Can you work these out from the model? Positions are in its coordinate system, mm. Face numbers are marked on the shaded views. A direction names the side the tool comes from. Round coordinates to 2 decimals unless told otherwise and drop trailing zeros. Loops run counter-clockwise (first coordinate to the right, second up) from the corner with the lowest first, then second, coordinate; pieces in that order, holes last. Notation, with made-up numbers: (82.25, -23.5) -> (111.25, -23.5) arc R34 cw to (111.25, 11.5) -> close; hole circle Ø4 at (-3.75, 80.25). An arc over 180 degrees is marked (long way). Write item = value, one per line.
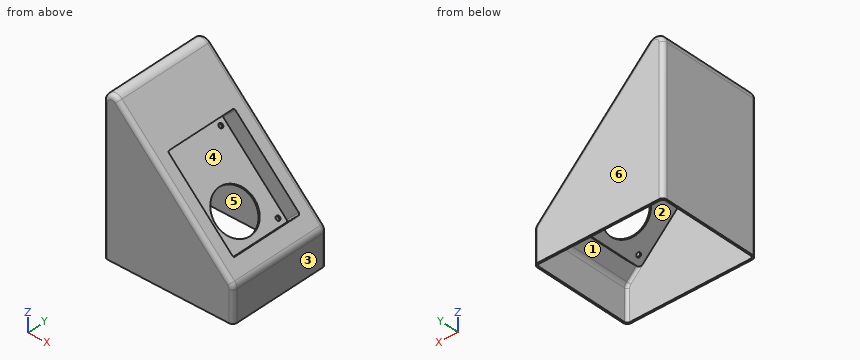
from build123d import *

# Parameters (mm, degrees)
F1_DEPTH = 60
F2_R     = 2.5
F2_R_2   = 25
F3_DEPTH = 20
F4_R     = 5
F5_T     = -2
F6_DEPTH = 25


with BuildPart() as f1:
    # F0 (on Front) → F1 (new body, symmetric)
    with BuildSketch(Plane.XZ):
        with BuildLine():
            Line((-84.0168925865, 63.0011496848), (-84.0168925865, -102.8567146915))
            Line((-84.0168925865, -102.8567146915), (65.9831074135, -102.8567146915))
            Line((65.9831074135, -102.8567146915), (65.9831074135, -66.9988503152))
            ThreePointArc((65.9831074135, -66.9988503152), (65.2219027386, -63.1720159916), (63.0541752254, -59.9277825033))
            Line((63.0541752254, -59.9277825033), (-66.9458247746, 70.0722174967))
            ThreePointArc((-66.9458247746, 70.0722174967), (-77.8437269101, 72.2399450099), (-84.0168925865, 63.0011496848))
        make_face()
    extrude(amount=F1_DEPTH, both=True)

    # F2 (on face) → F3 (cut)
    with BuildSketch(Plane(origin=(1.563196361, 0, 1.563196361), x_dir=(0.7071067812, 0, -0.7071067812), z_dir=(0.7071067812, 0, 0.7071067812))):
        with BuildLine():
            ThreePointArc((69.6613762736, 40.7), (69.0755898359, 42.1142135624), (67.6613762736, 42.7))
            Line((67.6613762736, 42.7), (-35.8386237264, 42.7))
            ThreePointArc((-35.8386237264, 42.7), (-37.2528372888, 42.1142135624), (-37.8386237264, 40.7))
            Line((-37.8386237264, 40.7), (-37.8386237264, -40.7))
            ThreePointArc((-37.8386237264, -40.7), (-37.2528372888, -42.1142135624), (-35.8386237264, -42.7))
            Line((-35.8386237264, -42.7), (67.6613762736, -42.7))
            ThreePointArc((67.6613762736, -42.7), (69.0755898359, -42.1142135624), (69.6613762736, -40.7))
            Line((69.6613762736, -40.7), (69.6613762736, 40.7))
        make_face()
        with Locations((-30.8386237264, -35.7)):
            Circle(F2_R, mode=Mode.SUBTRACT)
        with Locations((62.6613762736, -35.7)):
            Circle(F2_R, mode=Mode.SUBTRACT)
        with Locations((-30.8386237264, 35.7)):
            Circle(F2_R, mode=Mode.SUBTRACT)
        with Locations((37.6613762736, 0)):
            Circle(F2_R_2, mode=Mode.SUBTRACT)
        with Locations((62.6613762736, 35.7)):
            Circle(F2_R, mode=Mode.SUBTRACT)
        with Locations((37.6613762736, 0)):
            Circle(F2_R_2)
        with Locations((-30.8386237264, 35.7)):
            Circle(F2_R)
        with Locations((62.6613762736, 35.7)):
            Circle(F2_R)
        with Locations((62.6613762736, -35.7)):
            Circle(F2_R)
        with Locations((-30.8386237264, -35.7)):
            Circle(F2_R)
    extrude(amount=-F3_DEPTH, mode=Mode.SUBTRACT)

    # F4
    f4_edges = [f1.edges().sort_by_distance(p)[0] for p in [
        (-1.945825, 60, 5.072217),
        (-1.945825, -60, 5.072217),
    ]]
    fillet(f4_edges, radius=F4_R)

    # F5
    f5_openings = [f1.faces().sort_by_distance(p)[0] for p in [
        (-9.016893, 0, -102.856715),
    ]]
    offset(amount=F5_T, openings=f5_openings, kind=Kind.INTERSECTION)

    # F2 (on face) → F6 (cut)
    with BuildSketch(Plane(origin=(1.563196361, 0, 1.563196361), x_dir=(0.7071067812, 0, -0.7071067812), z_dir=(0.7071067812, 0, 0.7071067812))):
        with Locations((37.6613762736, 0)):
            Circle(F2_R_2)
        with Locations((-30.8386237264, 35.7)):
            Circle(F2_R)
        with Locations((-30.8386237264, -35.7)):
            Circle(F2_R)
        with Locations((62.6613762736, 35.7)):
            Circle(F2_R)
        with Locations((62.6613762736, -35.7)):
            Circle(F2_R)
    extrude(amount=-F6_DEPTH, mode=Mode.SUBTRACT)


solid = f1.part
1. I'm going to push flat-ended pins straight in: pin 1 (5 mm diameter, centred on x = -21.5, y = -11, fed in from +Z); pin 2 (3 mm diameter, centred on x = -63, y = -18, fed in from -Z); pin 3 (2 mm diameter, centred on x = -44, y = 30, fed in from -Z). Where does each tip first touch, or does it pass through?
Entries:
pin_1 = -1.16
pin_2 = 61.8
pin_3 = 43.3
2. For the marked faces 5 and 6, which set-ups out of +Z, -Z, +X, -X, +Y, -Y let a thin tool reach every point of the face, with its end or its side?
Entries:
face_5 = -Z
face_6 = +Z, -Z, +X, -X, +Y
3. Suppose I cut it at B-B, the plane y = 50. List the corners of the cut face in (x, z) for me.
Entries:
outline = (-84.02, -102.86) -> (-82.02, -102.86) -> (-82.02, 63) arc R8 cw to (-68.36, 68.66) -> (61.64, -61.34) arc R8 cw to (63.98, -67) -> (63.98, -102.86) -> (65.98, -102.86) -> (65.98, -67) arc R10 ccw to (63.05, -59.93) -> (-66.95, 70.07) arc R10 ccw to (-84.02, 63) -> close
4. I need wall thicknesses on line 1 (Y direction, x = -72, z = -77); line 2 (X direction, y = -36, z = 41); line 3 (Y direction, x = -17, z = -2). Which ranges of each line are inside material? Lowest first, please. Write a range as [from, to].
Entries:
line_1 = [-60, -58], [58, 60]
line_2 = [-84.02, -82.02], [-40.7, -37.87]
line_3 = [-60, -58], [-44.7, -42.7], [42.7, 44.7], [58, 60]
5. Suppose I cut it at A-A, the plane z = -78.5. List the corners of the cut face in (x, y) for me.
Entries:
outline = (-84.02, -55) arc R5 ccw to (-79.02, -60) -> (60.98, -60) arc R5 ccw to (65.98, -55) -> (65.98, 55) arc R5 ccw to (60.98, 60) -> (-79.02, 60) arc R5 ccw to (-84.02, 55) -> close; hole (-82.02, -55) arc R3 ccw to (-79.02, -58) -> (60.98, -58) arc R3 ccw to (63.98, -55) -> (63.98, 55) arc R3 ccw to (60.98, 58) -> (-79.02, 58) arc R3 ccw to (-82.02, 55) -> close
6. We'd pull the mould along Z, two halves only. Please class the marked faces 1, 2, 3 and 4: released by +Z, released by -Z, zero draft, split by the parting line, or undercut.
Entries:
face_1 = undercut
face_2 = released by -Z
face_3 = zero draft
face_4 = undercut
